Part model, mm, in its own coordinate system. A direction names the side the tool comes from. Coordinates: 2 decimals unless noted, no trailing zeros. Order: outer loops, then holes, each group sorted by start corner. A loop starts at its lowest first (then second) coordinate and runs counter-clockwise, first axis right, second up.
1) Pin check, flat tips, straight feed: pin 1 Ø1.5 at (y, z) = (0.5, -16.5) entering from +X; pin 2 Ø2 at (x, z) = (1, -15.5) entering from -Y. Stop position of each tip, or through.
2) Cut at A-A (z = -12.5). List the corners of the cut face in (x, y).
3) Tool access for faces 1 (the flat face through (0, 0, 8)), 2 (the flat face through (1.3, -1.3, 6)): list every direction of +Z, -Z, +X, -X, +Y, -Y with a clear straight run to the whole face (end or side of a thin tool).
4) Wall check: L1, parallel to X at y = 0, z = -7; L2, parallel to Z at x = -1.25, y = -1.25. Give the ranges that are in metal, low to high.
Autodesk Inventor part; units mm, degrees
ref_plane "YZ Plane" through (0, 0, 0) normal (1, 0, 0) x (0, 1, 0)
ref_plane "XZ Plane" through (0, 0, 0) normal (0, 1, 0) x (-1, 0, 0)
ref_plane "XY Plane" through (0, 0, 0) normal (0, 0, 1) x (1, 0, 0)
sketch "スケッチ1" plane through (0, 0, 0) normal (0, 0, 1) x (1, 0, 0)
  circle A0 centre (0, 0) radius 1.5
  dimension "d0" = 3
extrude "押し出し1" add sketch "スケッチ1" along normal blind 6
sketch "スケッチ2" plane through (0, 0, 6) normal (0, 0, 1) x (1, 0, 0)
  circle A0 centre (0, 0) radius 1.5
  circle A1 centre (0, 0) radius 3
  dimension "d3" = 6
extrude "押し出し2" add sketch "スケッチ2" along normal blind 2 contours A0 | A1
fillet "フィレット1" radius 2 1 edges at (-3, 0, 8)
thread "ねじ1"
sketch "スケッチ3" plane through (0, 0, 0) normal (0, 0, -1) x (-1, 0, 0)
  circle A0 centre (0, 0) radius 1.5
extrude "押し出し3" add sketch "スケッチ3" along normal blind 9
sketch "スケッチ4" plane through (0, 0, -9) normal (0, 0, -1) x (-1, 0, 0)
  circle A0 centre (0, 0) radius 1.5
extrude "押し出し4" add sketch "スケッチ4" along normal blind 5
sketch "スケッチ5" plane through (0, 0, -14) normal (0, 0, -1) x (-1, 0, 0)
  circle A0 centre (0, 0) radius 1.5
  dimension "d13" = 3
extrude "押し出し5" add sketch "スケッチ5" along normal blind 10
properties part number "SB　30mmなべネジ" material "Steel, Mild"
Geometry check:
1. pin 1: stops at x = 1.5
1. pin 2: stops at y = -1.5
2. outline: circle Ø3 at (0, 0)
3. face 1: +Z, +X, -X, +Y, -Y
3. face 2: -Z
4. L1: x = -1.5 to 1.5
4. L2: z = 6 to 7.85
